from build123d import *

# Parameters (mm, degrees)
BOSS_EXTRUDE1_DEPTH      = 20
BOSS_EXTRUDE1_DEPTH_BACK = 50
SKETCH4_W                = 5
SKETCH4_H                = 3
CUT_EXTRUDE1_DEPTH       = 25
CUT_EXTRUDE5_DEPTH       = 56
SKETCH10_W               = 35
SKETCH10_H               = 30
BOSS_EXTRUDE2_DEPTH      = 25
SKETCH13_W               = 9.28125
SKETCH13_H               = 5.15625
CUT_EXTRUDE6_DEPTH       = 25
SKETCH16_W               = 4
SKETCH16_H               = 8
BOSS_EXTRUDE4_DEPTH      = 6.2
SKETCH11_W               = 10
SKETCH11_H               = 10
CUT_EXTRUDE7_DEPTH       = 2


with BuildPart() as part:
    # Sketch1 → Boss-Extrude1 (new, two sides: drawn at the far end of the back side and taken through both)
    with BuildSketch(Plane.XY.offset(-BOSS_EXTRUDE1_DEPTH_BACK)):
        Polygon((-19.25, -26.5), (-11.25, -26.5), (-11.25, 26.5), (11.202, 26.5), (11.202, -26.5), (19.202, -26.5), (19.202, 34.5), (-19.25, 34.5), align=None)
    extrude(amount=BOSS_EXTRUDE1_DEPTH + BOSS_EXTRUDE1_DEPTH_BACK)

    # Sketch4 → Cut-Extrude1 (cut, symmetric)
    with BuildSketch(Plane(origin=(0, 31.309460855, 0), x_dir=(1, 0, 0), z_dir=(0, 1, 0))):
        with Locations((0, -9.645390894)):
            Rectangle(SKETCH4_W, SKETCH4_H)
    extrude(amount=CUT_EXTRUDE1_DEPTH, both=True, mode=Mode.SUBTRACT)

    # Sketch9 → Cut-Extrude5 (cut)
    with BuildSketch(Plane.XZ.offset(26.5)):
        Polygon((-15.25, -45.893834316), (15.202, -45.893834316), (15.202, -42.098185739), (21.427419281, -42.098185739), (21.427419281, -35.893834316), (15.202, -35.893834316), (-15.25, -35.893834316), (-21.646518422, -35.893834316), (-21.646518422, -42.093834316), (-15.25, -42.093834316), align=None)
    extrude(amount=-CUT_EXTRUDE5_DEPTH, mode=Mode.SUBTRACT)

    # Sketch10 → Boss-Extrude2 (add)
    with BuildSketch(Plane.ZY.offset(-11.202)):
        with Locations((-18.393834316, -11.5)):
            Rectangle(SKETCH10_W, SKETCH10_H)
    extrude(amount=BOSS_EXTRUDE2_DEPTH)

    # Sketch13 → Cut-Extrude6 (cut)
    with BuildSketch(Plane(origin=(0, 34.5, 0), x_dir=(1, 0, 0), z_dir=(0, 1, 0))):
        with Locations((-0.003125, 39.971959316)):
            Rectangle(SKETCH13_W, SKETCH13_H)
    extrude(amount=-CUT_EXTRUDE6_DEPTH, mode=Mode.SUBTRACT)

    # Sketch16 → Boss-Extrude4 (add)
    with BuildSketch(Plane.XY.offset(-42.093834316)):
        with Locations((-17.25, 25.5)):
            Rectangle(SKETCH16_W, SKETCH16_H)
        with Locations((17.202, 25.5)):
            Rectangle(SKETCH16_W, SKETCH16_H)
    extrude(amount=BOSS_EXTRUDE4_DEPTH)

    # Sketch11 → Cut-Extrude7 (cut)
    with BuildSketch(Plane.XY.offset(-0.893834316)):
        with Locations((-0.041292147, -15.960614003)):
            Rectangle(SKETCH11_W, SKETCH11_H)
    extrude(amount=-CUT_EXTRUDE7_DEPTH, mode=Mode.SUBTRACT)


solid = part.part
The model under review builds one solid part; all positions refer to its coordinate system, in mm. A direction names the side the tool comes from. Give positions to 0.01 mm unless a question says otherwise; leave off trailing zeros. Order: outer loops, then holes, each group sorted by start corner. A loop starts at its lowest first (then second) coordinate and runs counter-clockwise, first axis right, second up. Notation, with made-up numbers: M 75,9 L 97,9 A11 ccw 97,17 Z; hole C -10,84.5 d11. An arc over 180 degrees is marked long. One line per question, with ' | ' between items. Start each with the question number.
1) Mouldability with a two-part tool opening along X and no side actions: class faces 1 (the face through (-19.25, 4, -15)), 2 (the face through (0, 26.5, -48)), 3 (the face through (-13, 4, 20)) as pulls with the +X half, pulls with the -X half, needs draft (parallel to the pull), parting line crosses it, or undercut.
2) Wall thickness on L1, parallel to Z at x = 0, y = 28; L2, parallel to X at y = 4, z = 3; L3, parallel to Y at x = -5, z = -31: over which ranges is each line inside the solid? List them lowest first. Write a range as from..to.
3) Consider section D-D, the plane x = -1.5. Give the boundary of the cut face in (y, z), then the cut area to 3 significant figures.
4) Consider section A-A, the plane y = 16.5. Give the boundary of the cut face in (x, z), then the cut area to 3 significant figures.
5) For faces 4 (the face through (4.638, 32, -40)), 5 (the face through (-17, 21.5, -39)), 6 (the face through (15.202, 1, -44)), 7 (the face through (-11.25, 6, -2)), list the 3-axis set-ups (+Z, -Z, +X, -X, +Y, -Y) from which the entire face can be reached by the end or side of a thin tool; tool diameter is ignored.
6) Clearance check with flat-ended pins moving along their axes: P1, Ø3, axis at x = -3, y = -12.5, coming from the -Z side; P2, Ø4.5, axis at x = 2, z = -48, coming from the -Y side; P3, Ø2, axis at x = -16.5, z = -38.5, coming from the -Y side. State where each tip first meets the part, or that it passes through.
7) Consider section B-B, the plane y = -1. Give the boundary of the cut face in (x, z), then the cut area to 3 significant figures.
8) Consider section C-C, the plane z = -25. Give the boundary of the cut face in (x, y), then the cut area to 3 significant figures.
Found:
1) face 1: pulls with the -X half | face 2: undercut | face 3: needs draft
2) L1: z = -50..-45.89, -35.89..8.15, 11.15..20 | L2: x = -19.25..-11.25, 11.2..19.2 | L3: y = -26.5..3.5, 26.5..34.5
3) outline: M -26.5,-35.89 L 3.5,-35.89 L 3.5,-0.89 L -10.96,-0.89 L -10.96,-2.89 L -20.96,-2.89 L -20.96,-0.89 L -26.5,-0.89 Z; M 26.5,-50 L 34.5,-50 L 34.5,-42.55 L 29.5,-42.55 L 29.5,-45.89 L 26.5,-45.89 Z; M 26.5,-35.89 L 29.5,-35.89 L 29.5,-37.39 L 34.5,-37.39 L 34.5,8.15 L 26.5,8.15 Z; M 26.5,11.15 L 34.5,11.15 L 34.5,20 L 26.5,20 Z | area: 1,510 mm²
4) outline: M -19.25,-50 L -11.25,-50 L -11.25,-45.89 L -15.25,-45.89 L -15.25,-42.09 L -19.25,-42.09 Z; M -19.25,-35.89 L -11.25,-35.89 L -11.25,20 L -19.25,20 Z; M 11.2,-50 L 19.2,-50 L 19.2,-42.1 L 15.2,-42.1 L 15.2,-45.89 L 11.2,-45.89 Z; M 11.2,-35.89 L 19.2,-35.89 L 19.2,20 L 11.2,20 Z | area: 990 mm²
5) face 4: +Y, -Y | face 5: +X, -X, -Y | face 6: -Y | face 7: +Z
6) P1: stops at z = -35.89 | P2: stops at y = 26.5 | P3: stops at y = 21.5
7) outline: M -19.25,-50 L -11.25,-50 L -11.25,-45.89 L -15.25,-45.89 L -15.25,-42.09 L -19.25,-42.09 Z; M -19.25,-35.89 L 19.2,-35.89 L 19.2,20 L 11.2,20 L 11.2,-0.89 L -11.25,-0.89 L -11.25,20 L -19.25,20 Z; M 11.2,-50 L 19.2,-50 L 19.2,-42.1 L 15.2,-42.1 L 15.2,-45.89 L 11.2,-45.89 Z | area: 1,780 mm²
8) outline: M -19.25,-26.5 L 19.2,-26.5 L 19.2,34.5 L -19.25,34.5 Z; hole M -11.25,3.5 L 11.2,3.5 L 11.2,26.5 L -11.25,26.5 Z | area: 1,830 mm²
